```python
from build123d import *

# Parameters (mm, degrees)
SKETCH1_R           = 80
BOSS_EXTRUDE1_DEPTH = 19
SKETCH2_R           = 20
CUT_EXTRUDE1_DEPTH  = 115.721401665
SKETCH3_R           = 8.271230521
CUT_EXTRUDE2_DEPTH  = 18.790391
CIRPATTERN1_START   = 0.209609427
CIRPATTERN1_DEPTH   = 18.790390573


# Read off the part's stored shape, not the designer's step: CirPattern1
with BuildPart() as part:
    # Sketch1 → Boss-Extrude1 (new body)
    with BuildSketch(Plane(origin=(0, 0, 0), x_dir=(1, 0, 0), z_dir=(0, 1, 0))):
        with Locations(Location((0, 0, 0), (0, 0, 270))):
            Circle(SKETCH1_R)
    extrude(amount=BOSS_EXTRUDE1_DEPTH)

    # Sketch2 → Cut-Extrude1 (cut, through all)
    with BuildSketch(Plane(origin=(0, 0, 0), x_dir=(1, 0, 0), z_dir=(0, 1, 0))):
        with Locations(Location((0, 0, 0), (0, 0, 270))):
            Circle(SKETCH2_R)
    extrude(amount=CUT_EXTRUDE1_DEPTH, mode=Mode.SUBTRACT)

    # Sketch3 → Cut-Extrude2 (cut)
    with BuildSketch(Plane(origin=(0, 19, 0), x_dir=(1, 0, 0), z_dir=(0, 1, 0))):
        with Locations((-16.536495709, 0)):
            Circle(SKETCH3_R)
    extrude(amount=-CUT_EXTRUDE2_DEPTH, mode=Mode.SUBTRACT)

    # CirPattern1 outline → CirPattern1 (cut)
    with BuildSketch(Plane(origin=(0, 0, 0), x_dir=(1, 0, 0), z_dir=(0, 1, 0)).offset(CIRPATTERN1_START)):
        with BuildLine():
            ThreePointArc((-18.294155142, -8.082319447), (-18.6670657, -7.992116481), (-19.035392096, -7.884717571))
            ThreePointArc((-19.035392096, -7.884717571), (-17.541711443, -17.541711443), (-7.884717571, -19.035392096))
            ThreePointArc((-7.884717571, -19.035392096), (0, -24.80772623), (7.884717571, -19.035392096))
            ThreePointArc((7.884717571, -19.035392096), (17.541711443, -17.541711443), (19.035392096, -7.884717571))
            ThreePointArc((19.035392096, -7.884717571), (24.80772623, 0), (19.035392096, 7.884717571))
            ThreePointArc((19.035392096, 7.884717571), (17.541711443, 17.541711443), (7.884717571, 19.035392096))
            ThreePointArc((7.884717571, 19.035392096), (0, 24.80772623), (-7.884717571, 19.035392096))
            ThreePointArc((-7.884717571, 19.035392096), (-17.541711443, 17.541711443), (-19.035392096, 7.884717571))
            ThreePointArc((-19.035392096, 7.884717571), (-18.6670657, 7.992116481), (-18.294155142, 8.082319447))
            ThreePointArc((-18.294155142, 8.082319447), (20, 0), (-18.294155142, -8.082319447))
        make_face()
    extrude(amount=CIRPATTERN1_DEPTH, mode=Mode.SUBTRACT)


solid = part.part
```
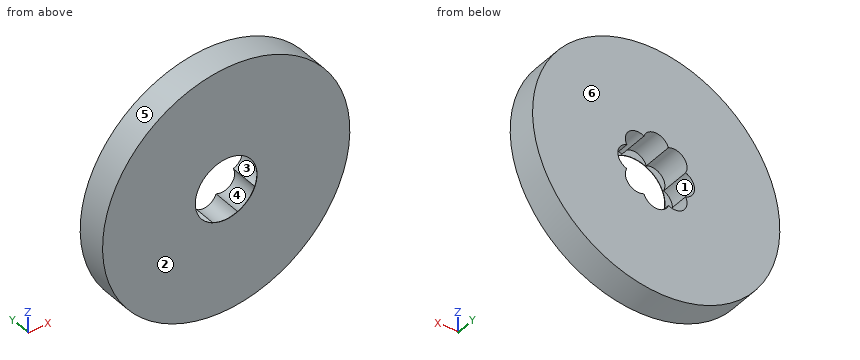
Read the model definition and answer for the solid it produces. Units are mm, in the model's axes. Face numbers are marked on the shaded views. A direction names the side the tool comes from. Give positions to 0.01 mm unless a question says otherwise; leave off trailing zeros. Loops run counter-clockwise (first coordinate to the right, second up) from the corner with the lowest first, then second, coordinate; pieces in that order, holes last.
Item 1: Each of these flat-tipped pins is pushed along its axis until it touches: pin 1 Ø5 at (x, z) = (-20.5, 1) entering from +Y; pin 2 Ø5 at (y, z) = (13, -62) entering from +X; pin 3 Ø24 at (x, z) = (0, 0) entering from -Y; pin 4 Ø1.5 at (y, z) = (8.5, 10) entering from -X. Where does it stop, or does it pass through?
Item 2: The part is cut by section B-B (z = 0). Write down the section's boundary in (x, y).
Item 3: The mould has two halves that part along Z. Classify the marked faces 3, 4, 5 and 6: released by +Z, released by -Z, zero draft, split by the parting line, or undercut.
Item 4: The part is cut by section C-C (y = 9.25). Write down the section's boundary in (x, z).
Item 5: The part is cut by section A-A (x = 0). Write down the section's boundary in (y, z).
Item 6: The part is cut by section D-D (z = -53). Write down the section's boundary in (x, y), and give its area (3 significant figures).
Item 7: Find the intervals of material crossed by line 1 along X through (y, z) = (0.15, 0); line 2 along X through (y, z) = (5.25, 23.5); line 3 along X through (y, z) = (14.75, 25), in increasing order.
Item 8: For the marked faces 1 and 2, determine the directions among +Z, -Z, +X, -X, +Y, -Y from which every point of the face is accessible in a straight line to the end or side of a thin tool.
Taken from the geometry:
1. pin 1: stops at y = 0.21
1. pin 2: stops at x = 53.48
1. pin 3: passes through
1. pin 4: stops at x = -79.46
2. outline: (-80, 0) - (-20, 0) - (-20, 0.21) - (-24.81, 0.21) - (-24.81, 19) - (-80, 19) - close; (20, 0) - (80, 0) - (80, 19) - (24.81, 19) - (24.81, 0.21) - (20, 0.21) - close
3. face 3: undercut
3. face 4: undercut
3. face 5: split by the parting line
3. face 6: zero draft
4. outline: circle Ø160 at (0, 0); hole (-19.04, -7.88) arc R8.27 ccw to (-7.88, -19.04) arc R8.27 ccw to (7.88, -19.04) arc R8.27 ccw to (19.04, -7.88) arc R8.27 ccw to (19.04, 7.88) arc R8.27 ccw to (7.88, 19.04) arc R8.27 ccw to (-7.88, 19.04) arc R8.27 ccw to (-19.04, 7.88) arc R8.27 ccw to start
5. outline: (0, -80) - (19, -80) - (19, -24.81) - (0.21, -24.81) - (0.21, -20) - (0, -20) - close; (0, 20) - (0.21, 20) - (0.21, 24.81) - (19, 24.81) - (19, 80) - (0, 80) - close
6. outline: (-59.92, 0) - (59.92, 0) - (59.92, 19) - (-59.92, 19) - close
6. area: 2,280 mm2
7. line 1: x = -80 to -20, 20 to 80
7. line 2: x = -76.47 to -4.46, 4.46 to 76.47
7. line 3: x = -75.99 to 75.99
8. face 1: +Y
8. face 2: +Z, -Z, +X, -X, -Y
